```python
from build123d import *

# Parameters (mm, degrees)
F0_R     = 1.5
F1_DEPTH = 4.8
F0_W     = 5
F0_H     = 4
F2_DEPTH = 2.8
F3_W     = 8
F3_H     = 6.4
F4_DEPTH = 4.701


with BuildPart() as f1:
    # F0 (on Front) → F1 (new body, symmetric)
    with BuildSketch(Plane.XZ):
        with BuildLine():
            Line((-13, -2), (-1.8138357147, -2))
            ThreePointArc((-1.8138357147, -2), (0.0723180492, -2.6990313262), (1.9183326093, -1.9))
            ThreePointArc((1.9183326093, -1.9), (2.7, 0), (1.9183326093, 1.9))
            ThreePointArc((1.9183326093, 1.9), (0.0723180492, 2.6990313262), (-1.8138357147, 2))
            Line((-1.8138357147, 2), (-13, 2))
            Line((-13, 2), (-13, -2))
        make_face()
        Circle(F0_R, mode=Mode.SUBTRACT)
    extrude(amount=F1_DEPTH, both=True)

    # F0 (on Front) → F2 (join, symmetric)
    with BuildSketch(Plane.XZ):
        with BuildLine():
            ThreePointArc((1.9183326093, 1.9), (2.7, 0), (1.9183326093, -1.9))
            Line((1.9183326093, -1.9), (13.3, -1.9))
            Line((13.3, -1.9), (13.3, 1.9))
            Line((13.3, 1.9), (1.9183326093, 1.9))
        make_face()
        with Locations((-15.5, 0)):
            Rectangle(F0_W, F0_H)
    extrude(amount=F2_DEPTH, both=True)

    # F3 (on face) → F4 (cut, through all)
    with BuildSketch(Plane.XY.offset(2)):
        with Locations((-6.2, 0)):
            Rectangle(F3_W, F3_H)
    extrude(amount=-F4_DEPTH, mode=Mode.SUBTRACT)


solid = f1.part
```
Check sheet for the modelled part. Datum: model origin and axes. Units: mm. A direction names the side the tool comes from. Round coordinates to 2 decimals unless told otherwise and drop trailing zeros. Loops run counter-clockwise (first coordinate to the right, second up) from the corner with the lowest first, then second, coordinate; pieces in that order, holes last. Notation, with made-up numbers: M 39,83.5 L 94,83.5 A18 ccw 94,107.5 Z; hole C 67.25,83 d8. An arc over 180 degrees is marked long. Answer as a JSON object with one key per item and string values.
1. Scan lines: line 1 (Y direction, x = -6.5, z = -0.4); line 2 (Z direction, x = 0, y = 2.5); line 3 (Z direction, x = 9, y = -2.5). Record each from-to range of solid material in increasing order.
Reply:
{"line 1": "y = -4.8 to -3.2, 3.2 to 4.8", "line 2": "z = -2.7 to -1.5, 1.5 to 2.7", "line 3": "z = -1.9 to 1.9"}
2. Access from +Z, -Z, +X, -X, +Y, -Y to the whole of each face (thin tool, end or side, straight path). Record for faces 1 (the flat face through (-6, 3.2, 0)), 2 (the flat face through (8, 0, -1.9)), 3 (the flat face through (-13, 4, 0)).
Reply:
{"face 1": "+Z, -Z", "face 2": "-Z, +X, +Y, -Y", "face 3": "+Z, -Z, -X, +Y"}
3. Mould release check, pull along X, two halves, no side actions. Record for faces 4 (the flat face through (-2.2, 0, 0)), 5 (the flat face through (-5, 4.8, 0)), 6 (the flat face through (-13, -4, 0)): pulls with the +X half, pulls with the -X half, needs draft (parallel to the pull), parting line crosses it, or undercut.
Reply:
{"face 4": "undercut", "face 5": "needs draft", "face 6": "pulls with the -X half"}
4. Section check C-C (x = 0). Record the boundary of the cut face in (y, z), plus the area to 3 significant figures.
Reply:
{"outline": "M -4.8,-2.7 L 4.8,-2.7 L 4.8,-1.5 L -4.8,-1.5 Z; M -4.8,1.5 L 4.8,1.5 L 4.8,2.7 L -4.8,2.7 Z", "area": "23.0 mm²"}
5. Gauge pin test, flat ends, axial feed: P1, Ø1.2, axis at x = -16.5, z = -0.5, coming from the -Y side; P2, Ø5, axis at x = -7.5, y = -1.5, coming from the +Z side; P3, Ø5, axis at x = -6.5, y = 1.5, coming from the -Z side. Record the tip position at first contact, or that the pin passes through.
Reply:
{"P1": "stops at y = -2.8", "P2": "stops at z = 2", "P3": "stops at z = -2"}
6. Section check D-D (y = 3.5). Record the boundary of the cut face in (x, z).
Reply:
{"outline": "M -13,-2 L -1.81,-2 A2.7 ccw long -1.81,2 L -13,2 Z; hole C 0,0 d3"}
7. Section check B-B (y = 0.5). Record the boundary of the cut face in (x, z).
Reply:
{"outline": "M -18,-2 L -10.2,-2 L -10.2,2 L -18,2 Z; M -2.2,-2 L -1.81,-2 A2.7 ccw 1.92,-1.9 L 13.3,-1.9 L 13.3,1.9 L 1.92,1.9 A2.7 ccw -1.81,2 L -2.2,2 Z; hole C 0,0 d3"}
8. Section check A-A (z = 0). Record the boundary of the cut face in (x, y), plus the area to 3 significant figures.
Reply:
{"outline": "M -18,-2.8 L -13,-2.8 L -13,-4.8 L -1.5,-4.8 L -1.5,4.8 L -13,4.8 L -13,2.8 L -18,2.8 Z; M 1.5,-4.8 L 2.7,-4.8 L 2.7,-2.8 L 13.3,-2.8 L 13.3,2.8 L 2.7,2.8 L 2.7,4.8 L 1.5,4.8 Z; hole M -10.2,-3.2 L -2.2,-3.2 L -2.2,3.2 L -10.2,3.2 Z", "area": "158 mm²"}
